Can you work these out from the model? Positions are in its coordinate system, mm. A direction names the side the tool comes from. Give positions to 0.01 mm unless a question says otherwise; leave off trailing zeros. Write each loop counter-clockwise with the first axis right and the second up, starting at its lowest first coordinate (ties: lowest second). Pieces come first, ordered by that corner, then holes. Notation, with made-up numbers: M -37.5,-6.75 L -14.5,-6.75 A24 ccw -14.5,20.25 Z; hole C -20.5,45 d6. An arc over 180 degrees is marked long. Write each question's results on one line, items separated by ' | '.
from build123d import *

# Parameters (mm, degrees)
SKETCH1_W           = 25.4
SKETCH1_H           = 15.24
BOSS_EXTRUDE1_DEPTH = 5.08
SKETCH2_R           = 1.651
CUT_EXTRUDE1_DEPTH  = 119.490202326
SKETCH3_W           = 12.7
SKETCH3_H           = 5.334
BOSS_EXTRUDE2_DEPTH = 52.578
SKETCH4_R           = 1.905
CUT_EXTRUDE2_DEPTH  = 115.262072587


with BuildPart() as part:
    # Sketch1 → Boss-Extrude1 (new body)
    with BuildSketch(Plane(origin=(0, 0, 0), x_dir=(1, 0, 0), z_dir=(0, 1, 0))):
        with Locations((-88.261608108, 54.193229454)):
            Rectangle(SKETCH1_W, SKETCH1_H)
    extrude(amount=-BOSS_EXTRUDE1_DEPTH)

    # Sketch2 → Cut-Extrude1 (cut, through all)
    with BuildSketch(Plane(origin=(0, 0, 0), x_dir=(1, 0, 0), z_dir=(0, 1, 0))):
        with Locations(Location((-94.611608108, 51.907229454, 0), (0, 0, 270))):
            Circle(SKETCH2_R)
        with Locations(Location((-81.911608108, 51.907229454, 0), (0, 0, 270))):
            Circle(SKETCH2_R)
    extrude(amount=-CUT_EXTRUDE1_DEPTH, mode=Mode.SUBTRACT)

    # Sketch3 → Boss-Extrude2 (add)
    with BuildSketch(Plane(origin=(0, 0, 0), x_dir=(1, 0, 0), z_dir=(0, 1, 0))):
        with Locations((-88.261608108, 59.146229454)):
            Rectangle(SKETCH3_W, SKETCH3_H)
    extrude(amount=BOSS_EXTRUDE2_DEPTH)

    # Sketch4 → Cut-Extrude2 (cut, through all)
    with BuildSketch(Plane.XY.offset(-56.479229454)):
        with Locations((-88.261608108, 46.228)):
            Circle(SKETCH4_R)
        with Locations((-88.261608108, 9.017)):
            Circle(SKETCH4_R)
    extrude(amount=-CUT_EXTRUDE2_DEPTH, mode=Mode.SUBTRACT)


solid = part.part
Item 1: If I drill on line 1 (Z direction, x = -88.5, y = 44); line 2 (Y direction, x = -80.5, z = -54); line 3 (X direction, y = 12, z = -59.5), over which ranges is the centre line in solid material (lowest first)? Write a range as from..to.
Geometry says:
line 1: z = -61.81..-56.48 | line 2: y = -5.08..0 | line 3: x = -94.61..-81.91
Item 2: I want a section at D-D, the plane y = 47. Please give me the cut outline in (x, z).
Geometry says:
outline: M -94.61,-61.81 L -90,-61.81 L -90,-56.48 L -94.61,-56.48 Z; M -86.52,-61.81 L -81.91,-61.81 L -81.91,-56.48 L -86.52,-56.48 Z
Item 3: Thinking about a two-plate mould opening in X: for faces 1 (the face through (-94.612, 26, -59)), 2 (the face through (-88, -3, -46.573)), 3 (the face through (-83.38, -2.5, -51.15)), which applies, +X half, -X half, draft (parallel to the pull), parting line (faces both ways), or undercut?
Geometry says:
face 1: -X half | face 2: draft | face 3: undercut
Item 4: I'm going to push flat-ended pins straight in: pin 1 (1 mm diameter, centred on y = 31, z = -59, fed in from +X); pin 2 (4.5 mm diameter, centred on x = -94.61, z = -51.91, fed in from +Y); pin 3 (8 mm diameter, centred on x = -95, y = 16, fed in from +Z). Where does each tip first touch, or does it pass through?
Geometry says:
pin 1: stops at x = -81.91 | pin 2: stops at y = 0 | pin 3: stops at z = -56.48
Item 5: I want a section at A-A, the plane y = -1. Please give me the cut outline in (x, z).
Geometry says:
outline: M -100.96,-61.81 L -75.56,-61.81 L -75.56,-46.57 L -100.96,-46.57 Z; hole C -94.61,-51.91 d3.3; hole C -81.91,-51.91 d3.3
Item 6: I want a section at C-C, the plane x = -88. Please give me the cut outline in (y, z).
Geometry says:
outline: M -5.08,-61.81 L 7.13,-61.81 L 7.13,-56.48 L 0,-56.48 L 0,-46.57 L -5.08,-46.57 Z; M 10.9,-61.81 L 44.34,-61.81 L 44.34,-56.48 L 10.9,-56.48 Z; M 48.11,-61.81 L 52.58,-61.81 L 52.58,-56.48 L 48.11,-56.48 Z
Item 7: I want a section at B-B, the plane z = -53. Please give me the cut outline in (x, y), and give its area (3 significant figures).
Geometry says:
outline: M -100.96,-5.08 L -95.85,-5.08 L -95.85,0 L -100.96,0 Z; M -93.37,-5.08 L -83.15,-5.08 L -83.15,0 L -93.37,0 Z; M -80.67,-5.08 L -75.56,-5.08 L -75.56,0 L -80.67,0 Z | area: 104 mm2
Item 8: For faces 4 (the face through (-81.912, 26, -59)), 5 (the face through (-88, 26, -56.479)), 6 (the face through (-88, 24, -61.813)), which set-ups out of +Z, -Z, +X, -X, +Y, -Y let a thin tool reach every point of the face, with its end or its side?
Geometry says:
face 4: +Z, -Z, +X, +Y | face 5: +Z, +X, -X, +Y | face 6: -Z, +X, -X, +Y, -Y
